Drawing for the job (mm, zero at the part's lowest x, y, z). A direction names the side the tool comes from. Give positions to 0.01 mm unless a question says otherwise; leave off trailing zeros. Write each loop counter-clockwise with the first axis right and the second up, starting at its lowest first coordinate (ties: lowest second). Pieces come first, ordered by that corner, then holes. Notation, with made-up numbers: M 65,82 L 78,82 A6 ccw 78,86 Z; hole C 48,-13 d9. An arc over 180 degrees is marked long. Use a Markdown table: item, result. Add a question column.
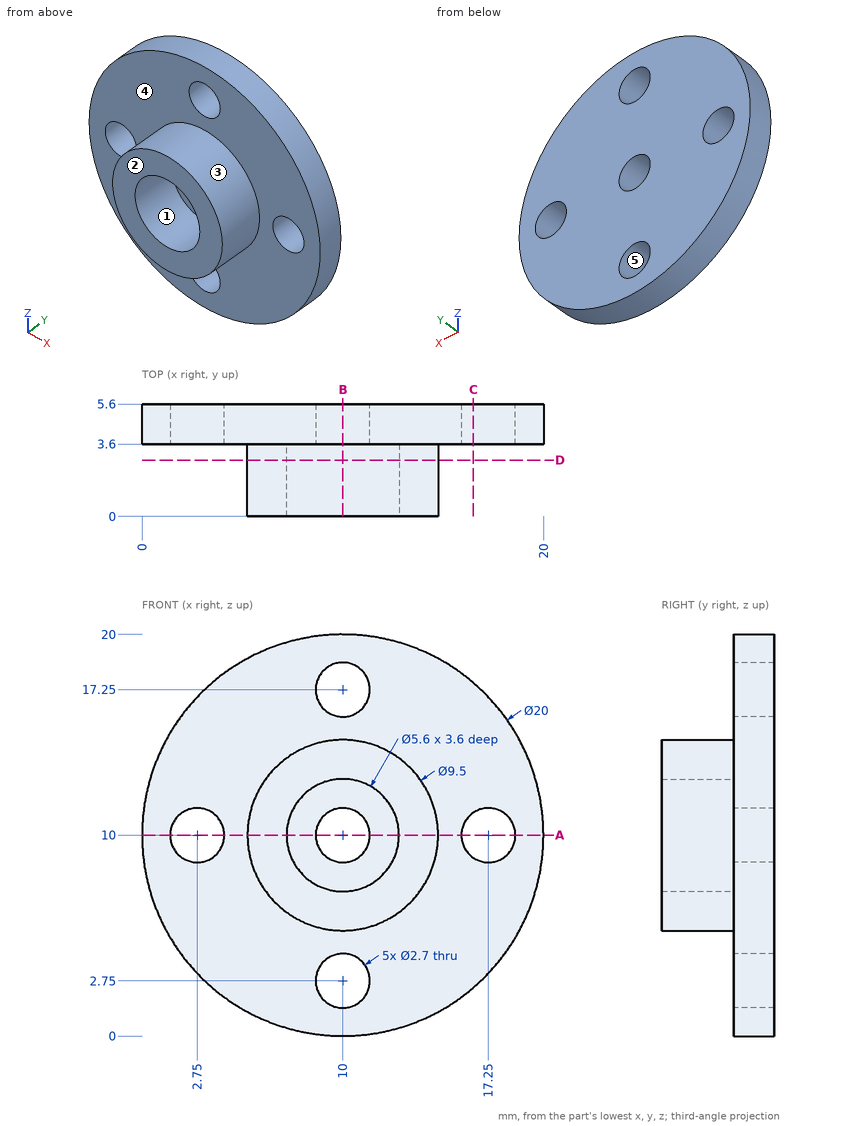
1. Cut at D-D (y = 2.8). Write the cut outline in (x, z), then the cut area to 3 significant figures.
2. Tool access for the marked faces 1 and 2: list every direction of +Z, -Z, +X, -X, +Y, -Y with a clear straight run to the whole face (end or side of a thin tool).
3. Cut at B-B (x = 10). Write the cut outline in (y, z), then the cut area to 3 significant figures.
4. Cut at A-A (z = 10). Write the cut outline in (x, y), then the cut area to 3 significant figures.
5. Flat gauge pins, fed straight in: pin 1 (1.5 mm diameter, centred on x = 15.5, y = 3, fed in from -Z); pin 2 (4.5 mm diameter, centred on x = 17.25, z = 10, fed in from -Y); pin 3 (1 mm diameter, centred on y = 1, z = 9.5, fed in from +X); pin 4 (2.5 mm diameter, centred on x = 10, z = 10, fed in from +Y). Where does each tip first touch, or does it go through?
6. Cut at C-C (x = 16.5). Write the cut outline in (y, z), then the cut area to 3 significant figures.
7. Mould opens along X. For the marked faces 3, 4 and 5 say: released by +X, released by -X, zero draft, split by the parting line, or undercut.
8. Drill centre lines: probe 1 along Z at (x, y) = (10, 4.15); probe 2 along Z at (x, y) = (10, 1.25); probe 3 along X at (y, z) = (5.35, 10.75). Where is each one in solid material? Low to high. Write a range as [from, to].
A:
| question | item | result |
|---|---|---|
| 1 | outline | C 10,10 d9.5; hole C 10,10 d5.6 |
| 1 | area | 46.3 mm² |
| 2 | face 1 | -Y |
| 2 | face 2 | +Z, -Z, +X, -X, -Y |
| 3 | outline | M 0,5.25 L 3.6,5.25 L 3.6,4.1 L 5.6,4.1 L 5.6,8.65 L 3.6,8.65 L 3.6,7.2 L 0,7.2 Z; M 0,12.8 L 3.6,12.8 L 3.6,11.35 L 5.6,11.35 L 5.6,15.9 L 3.6,15.9 L 3.6,14.75 L 0,14.75 Z; M 3.6,0 L 5.6,0 L 5.6,1.4 L 3.6,1.4 Z; M 3.6,18.6 L 5.6,18.6 L 5.6,20 L 3.6,20 Z |
| 3 | area | 37.8 mm² |
| 4 | outline | M 0,3.6 L 1.4,3.6 L 1.4,5.6 L 0,5.6 Z; M 4.1,3.6 L 5.25,3.6 L 5.25,0 L 7.2,0 L 7.2,3.6 L 8.65,3.6 L 8.65,5.6 L 4.1,5.6 Z; M 11.35,3.6 L 12.8,3.6 L 12.8,0 L 14.75,0 L 14.75,3.6 L 15.9,3.6 L 15.9,5.6 L 11.35,5.6 Z; M 18.6,3.6 L 20,3.6 L 20,5.6 L 18.6,5.6 Z |
| 4 | area | 37.8 mm² |
| 5 | pin 1 | stops at z = 1.37 |
| 5 | pin 2 | stops at y = 3.6 |
| 5 | pin 3 | stops at x = 14.75 |
| 5 | pin 4 | passes through |
| 6 | outline | M 3.6,2.4 L 5.6,2.4 L 5.6,8.88 L 3.6,8.88 Z; M 3.6,11.12 L 5.6,11.12 L 5.6,17.6 L 3.6,17.6 Z |
| 6 | area | 25.9 mm² |
| 7 | face 3 | split by the parting line |
| 7 | face 4 | zero draft |
| 7 | face 5 | undercut |
| 8 | probe 1 | z = [0, 1.4], [4.1, 8.65], [11.35, 15.9], [18.6, 20] |
| 8 | probe 2 | z = [5.25, 7.2], [12.8, 14.75] |
| 8 | probe 3 | x = [0.03, 1.63], [3.87, 8.88], [11.12, 16.13], [18.37, 19.97] |
